from build123d import *

# Parameters (mm, degrees)
F0_R     = 20
F1_DEPTH = 6
F2_DEPTH = 4.25
F3_R     = 12.75
F4_DEPTH = 5.5
F5_R     = 12
F6_DEPTH = 4.25
F7_R     = 5
F8_DEPTH = 73
F9_DEPTH = 20.001


# Not quite as in the source:
# - an extrude ends at something that could not be found from the text; its depth is read off the source's solid


with BuildPart() as f1:
    # F0 (on Top) → F1 (new body)
    with BuildSketch(Plane.XY):
        Circle(F0_R)
    extrude(amount=F1_DEPTH)

    # F2 (add): a face of the model
    f2_faces = [f1.faces().sort_by_distance(p)[0] for p in [
        (0, 0, 6),
    ]]
    extrude(f2_faces, amount=F2_DEPTH)

    # F3 (on face) → F4 (join)
    with BuildSketch(Plane.XY.offset(10.25)):
        Circle(F3_R)
    extrude(amount=F4_DEPTH)

    # F5 (on face) → F6 (join)
    with BuildSketch(Plane.XY.offset(15.75)):
        Circle(F5_R)
    extrude(amount=F6_DEPTH)

    # F7 (on face) → F8 (cut, through all)
    with BuildSketch(Plane.XY.offset(20)):
        Circle(F7_R)
    extrude(amount=F8_DEPTH, mode=Mode.SUBTRACT)

    # F7 (on face) → F9 (cut, through all)
    with BuildSketch(Plane.XY.offset(20)):
        Circle(F7_R)
    extrude(amount=-F9_DEPTH, mode=Mode.SUBTRACT)


solid = f1.part
Could you check a few things on this model? Use its own coordinates, in mm. A direction names the side the tool comes from. Round coordinates to 2 decimals unless told otherwise and drop trailing zeros. Order: outer loops, then holes, each group sorted by start corner. A loop starts at its lowest first (then second) coordinate and runs counter-clockwise, first axis right, second up.
Q1. I'm going to push flat-ended pins straight in: P1, Ø12, axis at y = -12, z = 9.5, coming from the -X side; P2, Ø9, axis at x = 0, y = 0, coming from the -Z side; P3, Ø1.5, axis at x = 11.5, z = 13, coming from the -Y side; P4, Ø1.5, axis at x = -10, z = 5, coming from the +Y side. Where does each tip first touch, or does it pass through?
Geometry says:
P1: stops at x = -19.08
P2: passes through
P3: stops at y = -6.86
P4: stops at y = 17.73
Q2. Thinking about a two-plate mould opening in X: for faces 3 (the face through (-1.08, -4.88, 10.14)), 4 (the face through (-2.764, -12.447, 12.962)), 5 (the face through (0, -13, 10.25)), which applies, released by +X, released by -X, zero draft, split by the parting line, or undercut?
Geometry says:
face 3: undercut
face 4: split by the parting line
face 5: zero draft
Q3. Imagine slicing it at C-C, the plane z = 2.25. List the corners of the cut face in (x, y) for me, then the cut area to 3 significant figures.
Geometry says:
outline: circle Ø40 at (0, 0); hole circle Ø10 at (0, 0)
area: 1,180 mm2
Q4. Please list where these lines run through material, in increasing order: probe 1 along Y at (x, z) = (0, 10); probe 2 along Z at (x, y) = (-9.5, 10.5); probe 3 along Y at (x, z) = (0, 15.5).
Geometry says:
probe 1: y = -20 to -5, 5 to 20
probe 2: z = 0 to 10.25
probe 3: y = -12.75 to -5, 5 to 12.75
Q5. Which directions (+Z, -Z, +X, -X, +Y, -Y) give clear straight access to the entire face, cutting with the end or side of a thin tool? Please do faces 1 (the face through (5.2, 0.2, 20)), 2 (the face through (-11.99, 0.53, 17.85)).
Geometry says:
face 1: +Z, +X, -X, +Y, -Y
face 2: +Z
Q6. Imagine slicing it at A-A, the plane x = 0. List the corners of the cut face in (y, z) for me, then the cut area to 3 significant figures.
Geometry says:
outline: (-20, 0) - (-5, 0) - (-5, 20) - (-12, 20) - (-12, 15.75) - (-12.75, 15.75) - (-12.75, 10.25) - (-20, 10.25) - close; (5, 0) - (20, 0) - (20, 10.25) - (12.75, 10.25) - (12.75, 15.75) - (12, 15.75) - (12, 20) - (5, 20) - close
area: 452 mm2
Q7. Imagine slicing it at D-D, the plane x = -16. List the corners of the cut face in (y, z) for me.
Geometry says:
outline: (-12, 0) - (12, 0) - (12, 10.25) - (-12, 10.25) - close
